from build123d import *

# Parameters (mm, degrees)
CROQUIS1_W              = 19.7
CROQUIS1_H              = 54.7
CROQUIS1_R              = 1.75
SALIENTE_EXTRUIR1_DEPTH = 3
CHAFL_N1_SIZE           = 0.6
CORTAR_EXTRUIR1_DEPTH   = 1.5
CROQUIS3_R              = 3.25
CORTAR_EXTRUIR2_DEPTH   = 30.224048316
SALIENTE_EXTRUIR2_DEPTH = 6


with BuildPart() as part:
    # Croquis1 → Saliente-Extruir1 (new body)
    with BuildSketch(Plane.XY):
        Rectangle(CROQUIS1_W, CROQUIS1_H)
        with Locations((-5, -24.35)):
            Circle(CROQUIS1_R, mode=Mode.SUBTRACT)
        with Locations((5, -24.35)):
            Circle(CROQUIS1_R, mode=Mode.SUBTRACT)
        with Locations(Location((5, 24.35, 0), (0, 0, 180))):
            Circle(CROQUIS1_R, mode=Mode.SUBTRACT)
        with Locations(Location((-5, 24.35, 0), (0, 0, 180))):
            Circle(CROQUIS1_R, mode=Mode.SUBTRACT)
    extrude(amount=SALIENTE_EXTRUIR1_DEPTH)

    # Chaflán1
    chafl_n1_edges = [part.edges().sort_by_distance(p)[0] for p in [
        (-6.75, -24.35, 0),
        (3.25, -24.35, 0),
        (6.75, 24.35, 0),
        (-3.25, 24.35, 0),
    ]]
    chamfer(chafl_n1_edges, length=CHAFL_N1_SIZE)

    # Croquis2 → Cortar-Extruir1 (cut)
    with BuildSketch(Plane.XY.offset(3)):
        Polygon((9.85, 20), (-9.85, 20), (-9.85, 17.5), (-7.85, 19), (7.85, 19), (9.85, 17.5), align=None)
        Polygon((-7.85, -19), (-9.85, -17.5), (-9.85, -20), (9.85, -20), (9.85, -17.5), (7.85, -19), align=None)
    extrude(amount=-CORTAR_EXTRUIR1_DEPTH, mode=Mode.SUBTRACT)

    # Croquis3 → Cortar-Extruir2 (cut, through all)
    with BuildSketch(Plane.XY.offset(3)):
        with Locations((0, 10.5)):
            Circle(CROQUIS3_R)
    extrude(amount=-CORTAR_EXTRUIR2_DEPTH, mode=Mode.SUBTRACT)

    # Croquis4 → Saliente-Extruir2 (add)
    with BuildSketch(Plane(origin=(0, 0, 0), x_dir=(-1, 0, 0), z_dir=(0, 0, -1))):
        Polygon((-9.85, -27.35), (-12.85, -27.35), (-12.85, 30.35), (9.85, 30.35), (9.85, 27.35), (-9.85, 27.35), align=None)
    extrude(amount=-SALIENTE_EXTRUIR2_DEPTH)


solid = part.part
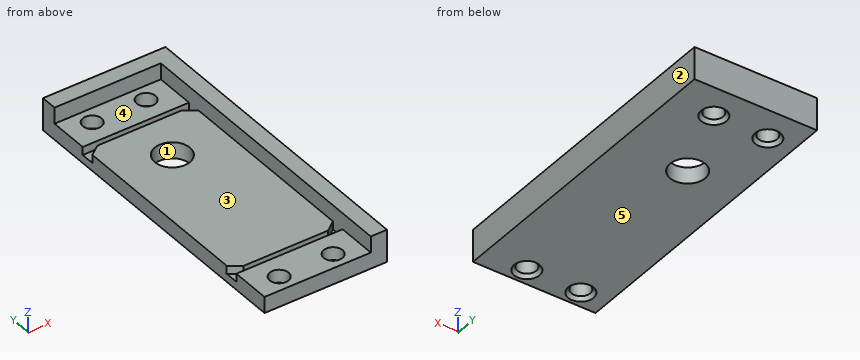
Read the model definition and answer for the solid it produces. Units are mm, in the model's axes. Face numbers are marked on the shaded views. A direction names the side the tool comes from. Round coordinates to 2 decimals unless told otherwise and drop trailing zeros. Loops run counter-clockwise (first coordinate to the right, second up) from the corner with the lowest first, then second, coordinate; pieces in that order, holes last.
Q1. Determine the mould class of the marked faces 1, 2 and 3 for opening direction X: released by +X, released by -X, zero draft, split by the parting line, or undercut.
Q2. Each of these flat-tipped pins is pushed along its axis until it touches: pin 1 (5 mm diameter, centred on x = -1.5, y = 13, fed in from -Z); pin 2 (4 mm diameter, centred on x = 5, y = -24.35, fed in from -Z); pin 3 (3 mm diameter, centred on x = -5, y = 24.35, fed in from -Z); pin 4 (2 mm diameter, centred on x = 8, z = 4.5, fed in from -Y). Where does it stop, or does it pass through?
Q3. Section B-B on z = 2.2 is taken. Write down the section's boundary in (x, y), and give its area (3 significant figures).
Q4. Which of the six approach directions +Z, -Z, +X, -X, +Y, -Y give full straight-line access (tool end or side, diameter ignored) to the marked faces 4 and 5?
Q5. Section D-D on y = -24.35 is taken. Write down the section's boundary in (x, z).
Q6. Section C-C on x = 0 is taken. Write down the section's boundary in (y, z), and give its area (3 significant figures).
Q7. Section A-A on y = 10.5 is taken. Write down the section's boundary in (x, z).
Q8. Consider probe 1 along Y at (x, z) = (-5, 1.65); probe 2 along Y at (x, z) = (-0.75, 1.75); probe 3 along X at (y, z) = (25, 5.7). Determine where each line is inside the solid, lowest interval first.
Output:
1. face 1: undercut
1. face 2: released by +X
1. face 3: zero draft
2. pin 1: stops at z = 0
2. pin 2: stops at z = 0.35
2. pin 3: passes through
2. pin 4: stops at y = 27.35
3. outline: (-9.85, -27.35) - (12.85, -27.35) - (12.85, 30.35) - (-9.85, 30.35) - (-9.85, 20) - (9.85, 20) - (9.85, 17.5) - (7.85, 19) - (-7.85, 19) - (-9.85, 17.5) - (-9.85, -17.5) - (-7.85, -19) - (7.85, -19) - (9.85, -17.5) - (9.85, -20) - (-9.85, -20) - close; hole circle Ø3.5 at (-5, -24.35); hole circle Ø3.5 at (-5, 24.35); hole circle Ø6.5 at (0, 10.5); hole circle Ø3.5 at (5, -24.35); hole circle Ø3.5 at (5, 24.35)
3. area: 1,190 mm2
4. face 4: +Z, -X, -Y
4. face 5: -Z, +X, -X, +Y, -Y
5. outline: (-9.85, 0) - (-7.35, 0) - (-6.75, 0.6) - (-6.75, 3) - (-9.85, 3) - close; (-3.25, 0.6) - (-2.65, 0) - (2.65, 0) - (3.25, 0.6) - (3.25, 3) - (-3.25, 3) - close; (6.75, 0.6) - (7.35, 0) - (12.85, 0) - (12.85, 6) - (9.85, 6) - (9.85, 3) - (6.75, 3) - close
6. outline: (-27.35, 0) - (7.25, 0) - (7.25, 3) - (-19, 3) - (-19, 1.5) - (-20, 1.5) - (-20, 3) - (-27.35, 3) - close; (13.75, 0) - (30.35, 0) - (30.35, 6) - (27.35, 6) - (27.35, 3) - (20, 3) - (20, 1.5) - (19, 1.5) - (19, 3) - (13.75, 3) - close
6. area: 160 mm2
7. outline: (-9.85, 0) - (-3.25, 0) - (-3.25, 3) - (-9.85, 3) - close; (3.25, 0) - (12.85, 0) - (12.85, 6) - (9.85, 6) - (9.85, 3) - (3.25, 3) - close
8. probe 1: y = -27.35 to -26.1, -22.6 to -20, -19 to 19, 20 to 22.6, 26.1 to 30.35
8. probe 2: y = -27.35 to -20, -19 to 7.34, 13.66 to 19, 20 to 30.35
8. probe 3: x = 9.85 to 12.85
